The listing builds one solid part. Answer for the finished solid, in the listing's coordinates (mm). A direction names the side the tool comes from. Coordinates: 2 decimals unless noted, no trailing zeros. Loops run counter-clockwise (first coordinate to the right, second up) from the corner with the lowest first, then second, coordinate; pieces in that order, holes last. Notation, with made-up numbers: M 16.25,83 L 49.25,83 A11 ccw 49.25,98 Z; hole C -31.5,-29.75 d7. An arc over 180 degrees is marked long. Answer as a JSON object with one key per item and string values. Group by question number.
1. Given pin 1 (1.9 mm diameter, centred on x = 0, y = 0, fed in from +Z); pin 2 (6 mm diameter, centred on y = 4.5, z = 11.5, fed in from -X); pin 3 (6 mm diameter, centred on y = -6.5, z = 11, fed in from +X); pin 4 (1.5 mm diameter, centred on y = 2.5, z = 10.5, fed in from +X), each flat-ended and moving along its own axis, determine where each tip first touches the part or whether it passes through.
2. For faces 1 (the face through (7, 0, 4)), 2 (the face through (-0.65, 1.01, 4.01)), determine the directions among +Z, -Z, +X, -X, +Y, -Y from which every point of the face is accessible in a straight line to the end or side of a thin tool.
3. A cutting plane is placed at A-A on y = 0. Give the vertices of the cut face in (x, z), and give its area (3 significant figures).
4. Straight lines are drawn through the part: L1, parallel to Y at x = 0, z = 3.55; L2, parallel to Y at x = 0, z = 4.15; L3, parallel to Z at x = -0.25, y = 8.75. For each, find the intervals that lie inside material, in ascending order.
5. Determine the mould class of faces 3 (the face through (-1.4, 4.5, 15)), 4 (the face through (-1.324, 0.417, 2.812)), 5 (the face through (6, 0, 9)) for opening direction Y: released by +Y, released by -Y, zero draft, split by the parting line, or undercut.
6. A cutting plane is placed at D-D on y = -8. Give the vertices of the cut face in (x, z), and give its area (3 significant figures).
7. A cutting plane is placed at C-C on z = 6.5. Give the vertices of the cut face in (x, y) (3 decimals).
from build123d import *

# Parameters (mm, degrees)
F2_SIZE = 3
F3_SIZE = 2


with BuildPart() as f1:
    # F0 (on Front) → F1 (revolve)
    with BuildSketch(Plane.XZ):
        Polygon((-1.2, 0), (-1.2, 5), (-2.2, 5), (-2.5, 15), (-6, 15), (-6, 4), (-10, 4), (-10, 0), align=None)
    revolve(axis=Axis((0, 0, 3.657732), (0, 0, -1)))

    # F2
    f2_edges = [f1.edges().sort_by_distance(p)[0] for p in [
        (1.2, 0, 0),
    ]]
    chamfer(f2_edges, length=F2_SIZE)

    # F3
    f3_edges = [f1.edges().sort_by_distance(p)[0] for p in [
        (2.5, 0, 15),
    ]]
    chamfer(f3_edges, length=F3_SIZE)


solid = f1.part
From the geometry:
{
 "1": {"pin 1": "passes through", "pin 2": "stops at x = -5.81", "pin 3": "stops at x = 4.87", "pin 4": "stops at x = 5.74"},
 "2": {"face 1": "+Z", "face 2": "+Z, -Z"},
 "3": {"outline": "M -10,0 L -4.2,0 L -1.2,3 L -1.2,5 L -2.2,5 L -2.44,13 L -4.5,15 L -6,15 L -6,4 L -10,4 Z; M 1.2,3 L 4.2,0 L 10,0 L 10,4 L 6,4 L 6,15 L 4.5,15 L 2.44,13 L 2.2,5 L 1.2,5 Z", "area": "140 mm²"},
 "4": {"L1": "y = -10 to -1.2, 1.2 to 10", "L2": "y = -6 to -1.2, 1.2 to 6", "L3": "z = 0 to 4"},
 "5": {"face 3": "zero draft", "face 4": "undercut", "face 5": "split by the parting line"},
 "6": {"outline": "M -6,0 L 6,0 L 6,4 L -6,4 Z", "area": "48.0 mm²"},
 "7": {"outline": "C 0,0 d12; hole C 0,0 d4.49"}
}
